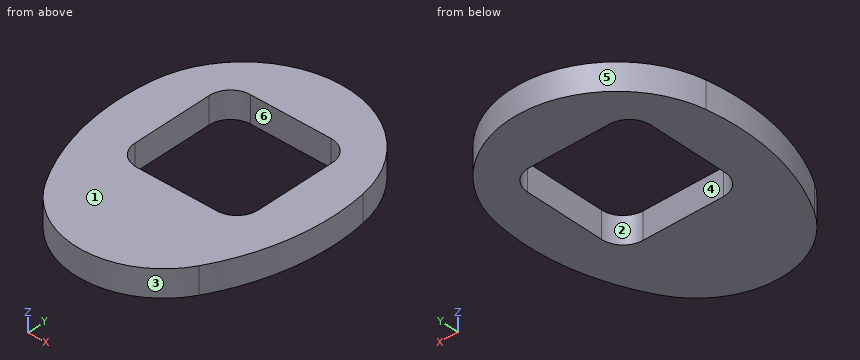
```python
from build123d import *

# Parameters (mm, degrees)
BOSS_EXTRUDE1_DEPTH = 6.35
CUT_EXTRUDE1_REACH  = 8.35
SKETCH2_W           = 29.21
SKETCH2_H           = 29.21
FILLET1_R           = 5.08


with BuildPart() as part:
    # Sketch1 → Boss-Extrude1 (new body)
    with BuildSketch(Plane.XY):
        with BuildLine():
            ThreePointArc((-24.784009304, 31.75), (-24.524700471, 13.689081607), (-18.172986801, -3.220080042))
            ThreePointArc((-18.172986801, -3.220080042), (0, -13.612941591), (18.172986801, -3.220080042))
            ThreePointArc((18.172986801, -3.220080042), (24.524700471, 13.689081607), (24.784009304, 31.75))
            ThreePointArc((24.784009304, 31.75), (0, 52.895043223), (-24.784009304, 31.75))
        make_face()
    extrude(amount=BOSS_EXTRUDE1_DEPTH)

    # Sketch2 → Cut-Extrude1 (cut, up to next)
    with BuildSketch(Plane.XY.offset(6.35), mode=Mode.PRIVATE) as cut_extrude1_sk1:
        with Locations((0, 25.4)):
            Rectangle(SKETCH2_W, SKETCH2_H)
    cut_extrude1_tool1 = extrude(cut_extrude1_sk1.sketch, amount=-CUT_EXTRUDE1_REACH, mode=Mode.PRIVATE) & part.part
    add(cut_extrude1_tool1.solids().sort_by_distance((0, 25.4, 6.35))[0], mode=Mode.SUBTRACT)

    # Fillet1
    fillet1_edges = [part.edges().sort_by_distance(p)[0] for p in [
        (14.605, 40.005, 3.175),
        (14.605, 10.795, 3.175),
        (-14.605, 10.795, 3.175),
        (-14.605, 40.005, 3.175),
    ]]
    fillet(fillet1_edges, radius=FILLET1_R)


solid = part.part
```
Verification items for the finished model (mm, model axes). Face numbers are marked on the shaded views. A direction names the side the tool comes from. Round coordinates to 2 decimals unless told otherwise and drop trailing zeros. Write each loop counter-clockwise with the first axis right and the second up, starting at its lowest first coordinate (ties: lowest second). Pieces come first, ordered by that corner, then holes. Notation, with made-up numbers: (6, -17.75) - (14, -17.75) arc R10 ccw to (14, -13.75) - close; hole circle Ø6 at (-13, -35). An arc over 180 degrees is marked (long way). Answer as a JSON object with one key per item and string values. Group by question number.
Q1. Mould release check, pull along X, two halves, no side actions. Record for the marked faces 1, 2, 3 and 4: released by +X, released by -X, zero draft, split by the parting line, or undercut.
Q2. Go/stop test with a flat-tipped pin: pin 1 Ø3 at (y, z) = (24, 4) entering from -X. Record where the tip stops, or that it passes through.
Q3. Tool access check on the marked faces 5 and 6. Record the directions out of +Z, -Z, +X, -X, +Y, -Y that give a thin tool (end or side, any length) a straight path to the whole face; none if there is none.
Q4. Section check B-B, the plane y = 29.5. Enter the section's corners in (x, z) (3 decimals), plus the area to 3 significant figures.
Q5. Section check D-D, the plane x = 15.5. Enter the section's corners in (y, z).
Q6. Section check A-A, the plane z = 1.25. Enter the section's corners in (x, y) (3 decimals), plus the area to 3 significant figures.
Q7. Section check C-C, the plane x = -2. Enter the section's corners in (y, z) (3 decimals), plus the area to 3 significant figures.
Q8. Thickness scan on line 1 (Y direction, x = -2, z = 1) (3 decimals); line 2 (X direction, y = 30, z = 5) (3 decimals); line 3 (X direction, y = 17.5, z = 1.5) (3 decimals). Record the ranges inside material, lowest first.
Found:
{
 "1": {"face 1": "zero draft", "face 2": "undercut", "face 3": "split by the parting line", "face 4": "undercut"},
 "2": {"pin 1": "stops at x = -25.44"},
 "3": {"face 5": "+Z, -Z, +Y", "face 6": "+Z, -Z"},
 "4": {"outline": "(-25.093, 0) - (-14.605, 0) - (-14.605, 6.35) - (-25.093, 6.35) - close; (14.605, 0) - (25.093, 0) - (25.093, 6.35) - (14.605, 6.35) - close", "area": "133 mm^2"},
 "5": {"outline": "(-6.82, 0) - (47.54, 0) - (47.54, 6.35) - (-6.82, 6.35) - close"},
 "6": {"outline": "(-24.784, 31.75) arc R52.621 ccw to (-18.173, -3.22) arc R21.085 ccw to (18.173, -3.22) arc R52.621 ccw to (24.784, 31.75) arc R25.097 ccw to start; hole (-14.605, 15.875) arc R5.08 ccw to (-9.525, 10.795) - (9.525, 10.795) arc R5.08 ccw to (14.605, 15.875) - (14.605, 34.925) arc R5.08 ccw to (9.525, 40.005) - (-9.525, 40.005) arc R5.08 ccw to (-14.605, 34.925) - close", "area": "1,880 mm^2"},
 "7": {"outline": "(-13.518, 0) - (10.795, 0) - (10.795, 6.35) - (-13.518, 6.35) - close; (40.005, 0) - (52.815, 0) - (52.815, 6.35) - (40.005, 6.35) - close", "area": "236 mm^2"},
 "8": {"line 1": "y = -13.518 to 10.795, 40.005 to 52.815", "line 2": "x = -25.033 to -14.605, 14.605 to 25.033", "line 3": "x = -25.101 to -14.605, 14.605 to 25.101"}
}
